The model under review builds one solid part; all positions refer to its coordinate system, in mm. Face numbers are marked on the shaded views. A direction names the side the tool comes from. Give positions to 0.01 mm unless a question says otherwise; leave off trailing zeros. Order: outer loops, then holes, each group sorted by start corner. A loop starts at its lowest first (then second) coordinate and runs counter-clockwise, first axis right, second up. Notation, with made-up numbers: (-34, 24.25) -> (5, 24.25) arc R12 ccw to (5, 33.25) -> close; hole circle Ø4 at (-27, 44). An arc over 180 degrees is marked (long way). Answer as a JSON object with one key per item and string values. Group by question number.
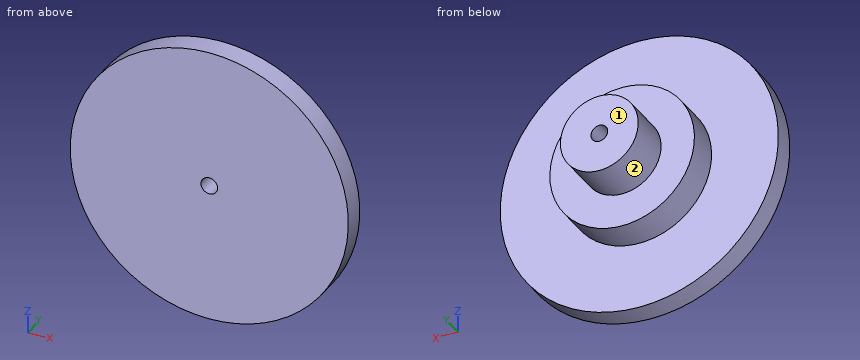
from build123d import *

# Parameters (mm, degrees)
SKETCH1_R           = 25
BOSS_EXTRUDE1_DEPTH = 4
SKETCH2_R           = 13
BOSS_EXTRUDE2_DEPTH = 6
SKETCH3_R           = 7
BOSS_EXTRUDE3_DEPTH = 8
SKETCH4_R           = 1.5
CUT_EXTRUDE1_DEPTH  = 40.67366885


with BuildPart() as part:
    # Sketch1 → Boss-Extrude1 (new body)
    with BuildSketch(Plane(origin=(0, 0, 0), x_dir=(1, 0, 0), z_dir=(0, 1, 0))):
        with Locations(Location((0, 0, 0), (0, 0, 270))):
            Circle(SKETCH1_R)
    extrude(amount=BOSS_EXTRUDE1_DEPTH)

    # Sketch2 → Boss-Extrude2 (add)
    with BuildSketch(Plane(origin=(0, 4, 0), x_dir=(1, 0, 0), z_dir=(0, 1, 0))):
        with Locations(Location((0, 0, 0), (0, 0, 270))):
            Circle(SKETCH2_R)
    extrude(amount=BOSS_EXTRUDE2_DEPTH)

    # Sketch3 → Boss-Extrude3 (add)
    with BuildSketch(Plane(origin=(0, 10, 0), x_dir=(1, 0, 0), z_dir=(0, 1, 0))):
        with Locations(Location((0, 0, 0), (0, 0, 270))):
            Circle(SKETCH3_R)
    extrude(amount=BOSS_EXTRUDE3_DEPTH)

    # Sketch4 → Cut-Extrude1 (cut, through all)
    with BuildSketch(Plane(origin=(0, 18, 0), x_dir=(1, 0, 0), z_dir=(0, 1, 0))):
        with Locations(Location((0, 0, 0), (0, 0, 270))):
            Circle(SKETCH4_R)
    extrude(amount=-CUT_EXTRUDE1_DEPTH, mode=Mode.SUBTRACT)


solid = part.part
1. Take a section at A-A on z = 0. Give the boundary of the cut face in (x, y).
2. Take a section at B-B on x = 0. Give the boundary of the cut face in (y, z).
3. For pin 1 (4 mm diameter, centred on x = -18, z = -7.5, fed in from +Y); pin 2 (6 mm diameter, centred on y = 7.5, z = 4, fed in from +X); pin 3 (4 mm diameter, centred on x = -1, y = 5.5, fed in from +Z); pin 4 (10 mm diameter, centred on x = 6, y = 7.5, fed in from +Z), all flat-tipped, find the tip position at first contact; note any pin that passes through.
4. Take a section at C-C on y = 11. Give the boundary of the cut face in (x, z), plus the area to 3 significant figures.
5. Take a section at D-D on z = -5.5. Give the boundary of the cut face in (x, y), plus the area to 3 significant figures.
6. For probe 1 along X at (y, z) = (10.25, 0); probe 2 along X at (y, z) = (6.5, 0); probe 3 along Y at (x, z) = (-0.5, 11.5), list the stretches that pass through material, from the lowest coordinate up. Write a range as [from, to].
7. Machinability: for the marked faces 1 and 2, which of the approach directions +Z, -Z, +X, -X, +Y, -Y give a long, thin tool a straight path to every point of the face, cutting with its end or side? Answer none if there is none.
Checks:
{
 "1": {"outline": "(-25, 0) -> (-1.5, 0) -> (-1.5, 18) -> (-7, 18) -> (-7, 10) -> (-13, 10) -> (-13, 4) -> (-25, 4) -> close; (1.5, 0) -> (25, 0) -> (25, 4) -> (13, 4) -> (13, 10) -> (7, 10) -> (7, 18) -> (1.5, 18) -> close"},
 "2": {"outline": "(0, -25) -> (4, -25) -> (4, -13) -> (10, -13) -> (10, -7) -> (18, -7) -> (18, -1.5) -> (0, -1.5) -> close; (0, 1.5) -> (18, 1.5) -> (18, 7) -> (10, 7) -> (10, 13) -> (4, 13) -> (4, 25) -> (0, 25) -> close"},
 "3": {"pin 1": "stops at y = 4", "pin 2": "stops at x = 12.96", "pin 3": "stops at z = 25", "pin 4": "stops at z = 24.88"},
 "4": {"outline": "circle Ø14 at (0, 0); hole circle Ø3 at (0, 0)", "area": "147 mm2"},
 "5": {"outline": "(-24.39, 0) -> (24.39, 0) -> (24.39, 4) -> (11.78, 4) -> (11.78, 10) -> (4.33, 10) -> (4.33, 18) -> (-4.33, 18) -> (-4.33, 10) -> (-11.78, 10) -> (-11.78, 4) -> (-24.39, 4) -> close", "area": "406 mm2"},
 "6": {"probe 1": "x = [-7, -1.5], [1.5, 7]", "probe 2": "x = [-13, -1.5], [1.5, 13]", "probe 3": "y = [0, 10]"},
 "7": {"face 1": "+Z, -Z, +X, -X, +Y", "face 2": "+Y"}
}
